Could you check a few things on this model? Use its own coordinates, in mm. A direction names the side the tool comes from. Give positions to 0.01 mm unless a question says otherwise; leave off trailing zeros. Loops run counter-clockwise (first coordinate to the right, second up) from the corner with the lowest first, then second, coordinate; pieces in that order, holes last. Notation, with made-up numbers: M -33.5,-33.5 L -1.5,-33.5 A31 ccw -1.5,-6.5 Z; hole C -39.75,-12.5 d8. An arc over 180 degrees is marked long. Use a Markdown table: item, result. Add a question column.
1) Suppose I cut it at C-C on z = 7.5. List the corners of the cut face in (x, y) for me (1 decimal), and give its area (3 significant figures).
2) If I drill on line 1 along Z through (x, y) = (-10, -26) (3 decimals); line 2 along Y through (x, z) = (0, 46); line 3 along Y through (x, z) = (-5.75, 33), over which ranges is the centre line in solid material (lowest first)? Write a range as [from, to].
3) Suppose I cut it at A-A on x = 0. List the corners of the cut face in (y, z) for me (1 decimal).
4) Which directions (+Z, -Z, +X, -X, +Y, -Y) give clear straight access to the entire face, cutting with the end or side of a thin tool? Please do faces 1 (the flat face through (0, -49.147, 26)), 2 (the cylindrical face through (0.259, 11.768, 45.971)).
5) Suppose I cut it at D-D on x = -7.75. List the corners of the cut face in (y, z) for me (3 decimals), and give its area (3 significant figures).
6) We'd pull the mould along Z, two halves only. Please class faces 3 (the flat face through (0, -22, 0)), 4 (the flat face through (0, -18, 41.275)), 5 (the flat face through (-11.771, -28, 8)): +Z half, -Z half, draft (parallel to the pull), parting line (faces both ways), or undercut.
7) Suppose I cut it at B-B on y = -6. List the corners of the cut face in (x, z) for me (3 decimals), and give its area (3 significant figures).
8) Will this pin go through, and if not, where does the flat tip stop? pin 1 Ø3 at (x, z) = (0, 11.5) entering from +Y.
```python
from build123d import *

# Parameters (mm, degrees)
F0_R     = 4.7625
F1_DEPTH = 50.8
F2_W     = 18.094934
F2_H     = 31.75
F3_DEPTH = 23.542328


with BuildPart() as f1:
    # F0 (on Top) → F1 (new body)
    with BuildSketch(Plane.XY):
        with BuildLine():
            Line((-11.770664, 0), (-11.770664, -56.734564))
            Line((-11.770664, -56.734564), (11.770664, -56.734564))
            Line((11.770664, -56.734564), (11.770664, 0))
            ThreePointArc((11.770664, 0), (0, 11.770664), (-11.770664, 0))
        make_face()
        Circle(F0_R, mode=Mode.SUBTRACT)
    extrude(amount=F1_DEPTH)

    # F2 (on face) → F3 (cut, through all)
    with BuildSketch(Plane.YZ.offset(11.770664)):
        Polygon((-35.73535, 41.275), (-49.146869, 41.275), (-49.146869, 9.525), (-35.73535, 9.525), (0, 9.525), (0, 41.275), align=None)
        with Locations((9.047467, 25.4)):
            Rectangle(F2_W, F2_H)
    extrude(amount=-F3_DEPTH, mode=Mode.SUBTRACT)


solid = f1.part
```
Answer block:
| question | item | result |
|---|---|---|
| 1 | outline | M -11.8,-56.7 L 11.8,-56.7 L 11.8,0 A11.8 ccw -11.8,0 Z; hole C 0,0 d9.5 |
| 1 | area | 1,480 mm^2 |
| 2 | line 1 | z = [0, 9.525], [41.275, 50.8] |
| 2 | line 2 | y = [-56.73, -4.76], [4.76, 11.77] |
| 2 | line 3 | y = [-56.73, -49.15] |
| 3 | outline | M -56.7,0 L -4.8,0 L -4.8,9.5 L -49.1,9.5 L -49.1,41.3 L -4.8,41.3 L -4.8,50.8 L -56.7,50.8 Z; M 4.8,0 L 11.8,0 L 11.8,9.5 L 4.8,9.5 Z; M 4.8,41.3 L 11.8,41.3 L 11.8,50.8 L 4.8,50.8 Z |
| 4 | face 1 | +X, -X, +Y |
| 4 | face 2 | +Z, -Z, +Y |
| 5 | outline | M -56.735,0 L 8.859,0 L 8.859,9.525 L -49.147,9.525 L -49.147,41.275 L 8.859,41.275 L 8.859,50.8 L -56.735,50.8 Z |
| 5 | area | 1,490 mm^2 |
| 6 | face 3 | -Z half |
| 6 | face 4 | undercut |
| 6 | face 5 | draft |
| 7 | outline | M -11.771,0 L 11.771,0 L 11.771,9.525 L -11.771,9.525 Z; M -11.771,41.275 L 11.771,41.275 L 11.771,50.8 L -11.771,50.8 Z |
| 7 | area | 448 mm^2 |
| 8 | pin 1 | stops at y = -49.15 |
